Geometry check sheet. Reference: the model listing, model coordinates, mm. Coordinates: 2 decimals unless noted, no trailing zeros. Order: outer loops, then holes, each group sorted by start corner. A loop starts at its lowest first (then second) coordinate and runs counter-clockwise, first axis right, second up. Notation, with made-up numbers: (41.25, 50.5) - (90.25, 50.5) arc R12 ccw to (90.25, 64.5) - close; hole circle Ø9 at (68, 40). An arc over 180 degrees is marked (long way). Put each result on its own line as item: value.
from build123d import *

# Parameters (mm, degrees)
SKETCH2_W             = 2
SKETCH2_H             = 12
CUT_EXTRUDE1_DEPTH    = 10
SKETCH4_R             = 1.25
CUT_EXTRUDE2_DEPTH    = 10
CRVPATTERN2_OUTLINE_R = 1.25
CRVPATTERN2_DEPTH     = 2
SKETCH7_R             = 1.6
CUT_EXTRUDE3_DEPTH    = 2
SKETCH8_R             = 1.6
CUT_EXTRUDE4_DEPTH    = 11


# Read off the part's stored shape, not the designer's step: CrvPattern2
with BuildPart() as part:
    # Sweep1: sweep along a path in Sketch1
    with BuildLine(Plane(origin=(0, 0, 0), x_dir=(0, 0, -1), z_dir=(1, 0, 0))) as sweep1_path:
        ThreePointArc((0, 163.5), (-72.196731601, 108.101499399), (-37.371778265, 24.026624746))
        ThreePointArc((-37.371778265, 24.026624746), (-27.216931784, 13.871778265), (-23.5, 0))
    # Sketch2 → Sweep1 (sweep)
    with BuildSketch(Plane(origin=(0, 0, 0), x_dir=(1, 0, 0), z_dir=(0, 1, 0))):
        with Locations((1, -29.5)):
            Rectangle(SKETCH2_W, SKETCH2_H)
    sweep(path=sweep1_path.line)

    # Sketch3 → Cut-Extrude1 (cut)
    with BuildSketch(Plane(origin=(2, 0, 0), x_dir=(0, 0, -1), z_dir=(1, 0, 0))):
        with BuildLine():
            Line((0, 88.75644347), (-15.062860516, 174.182170465))
            ThreePointArc((-15.062860516, 174.182170465), (-7.560199098, 175.169914579), (0, 175.5))
            Line((0, 175.5), (0, 88.75644347))
        make_face()
    extrude(amount=-CUT_EXTRUDE1_DEPTH, mode=Mode.SUBTRACT)

    # Sketch4 → Cut-Extrude2 (cut)
    with BuildSketch(Plane.ZY):
        with Locations((26.912638139, 4.5)):
            Circle(SKETCH4_R)
    extrude(amount=-CUT_EXTRUDE2_DEPTH, mode=Mode.SUBTRACT)

    # CrvPattern2 outline → CrvPattern2 (cut)
    with BuildSketch(Plane.YZ):
        with Locations((18.911112769, 35.286946502)):
            Circle(CRVPATTERN2_OUTLINE_R)
        with Locations((12.43190695, 29.849835971)):
            Circle(CRVPATTERN2_OUTLINE_R)
        with Locations((161.000106646, 28.721311128)):
            Circle(CRVPATTERN2_OUTLINE_R)
        with Locations((157.434782313, 36.432764864)):
            Circle(CRVPATTERN2_OUTLINE_R)
        with Locations((153.049302567, 43.709139217)):
            Circle(CRVPATTERN2_OUTLINE_R)
        with Locations((147.896038722, 50.463539862)):
            Circle(CRVPATTERN2_OUTLINE_R)
        with Locations((142.036530957, 56.615305875)):
            Circle(CRVPATTERN2_OUTLINE_R)
        with Locations((135.540753402, 62.090972984)):
            Circle(CRVPATTERN2_OUTLINE_R)
        with Locations((128.486278509, 66.825150876)):
            Circle(CRVPATTERN2_OUTLINE_R)
        with Locations((120.957350684, 70.76130409)):
            Circle(CRVPATTERN2_OUTLINE_R)
        with Locations((113.043880237, 73.852427158)):
            Circle(CRVPATTERN2_OUTLINE_R)
        with Locations((104.840369684, 76.061605948)):
            Circle(CRVPATTERN2_OUTLINE_R)
        with Locations((96.44478519, 77.362458489)):
            Circle(CRVPATTERN2_OUTLINE_R)
        with Locations((87.957386665, 77.739450025)):
            Circle(CRVPATTERN2_OUTLINE_R)
        with Locations((79.479530462, 77.188078529)):
            Circle(CRVPATTERN2_OUTLINE_R)
        with Locations((71.112458978, 75.714928469)):
            Circle(CRVPATTERN2_OUTLINE_R)
        with Locations((62.956091619, 73.337592177)):
            Circle(CRVPATTERN2_OUTLINE_R)
        with Locations((55.107831572, 70.084459755)):
            Circle(CRVPATTERN2_OUTLINE_R)
        with Locations((47.661402606, 65.994380051)):
            Circle(CRVPATTERN2_OUTLINE_R)
        with Locations((40.705729836, 61.116196717)):
            Circle(CRVPATTERN2_OUTLINE_R)
        with Locations((34.323877772, 55.508164926)):
            Circle(CRVPATTERN2_OUTLINE_R)
        with Locations((28.592058371, 49.237255687)):
            Circle(CRVPATTERN2_OUTLINE_R)
        with Locations((23.578720911, 42.378356079)):
            Circle(CRVPATTERN2_OUTLINE_R)
    extrude(amount=CRVPATTERN2_DEPTH, mode=Mode.SUBTRACT)

    # Sketch7 → Cut-Extrude3 (cut)
    with BuildSketch(Plane.ZY):
        with Locations((35.390452374, 10)):
            Circle(SKETCH7_R)
        with Locations((76.299174561, 54.239502389)):
            Circle(SKETCH7_R)
        with Locations((79.721620809, 114.397161787)):
            Circle(SKETCH7_R)
        with Locations((41.871778265, 161.280490828)):
            Circle(SKETCH7_R)
    extrude(amount=-CUT_EXTRUDE3_DEPTH, mode=Mode.SUBTRACT)

    # Sketch8 → Cut-Extrude4 (cut)
    with BuildSketch(Plane(origin=(2, 0, 0), x_dir=(0, 0, -1), z_dir=(1, 0, 0))):
        with Locations((-19.266049694, 169.225788418)):
            Circle(SKETCH8_R)
    extrude(amount=-CUT_EXTRUDE4_DEPTH, mode=Mode.SUBTRACT)


solid = part.part
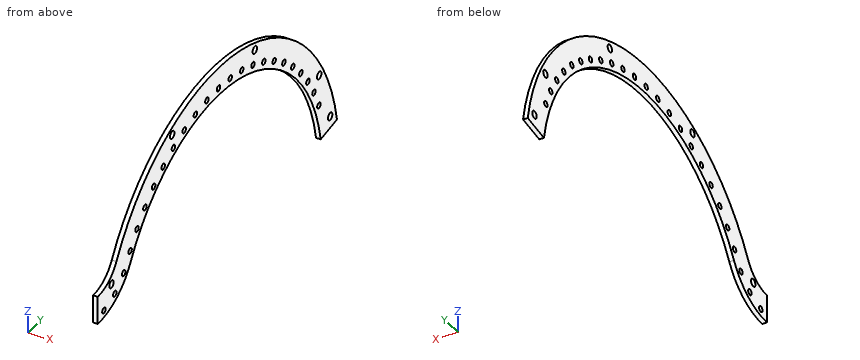
Q1. Section check B-B on x = 1.05. State how many separate pieces and enclosed holes the cut face has, then the cut area to 3 significant figures.
Answer block:
separate pieces: 1
enclosed holes: 29
area: 2,480 mm^2
Q2. Depth check by flat-ended pin: pin 1 Ø1 at (x, y) = (1.5, 65.5) entering from -Z. Enter the tip coordinate at first touch or a pass-through.
Answer block:
pin 1: stops at z = 70.87
Q3. Section check A-A on y = 100. Record the boundary of the cut face in (x, z), then the cut area to 3 significant figures.
Answer block:
outline: (0, 73.89) - (2, 73.89) - (2, 86.01) - (0, 86.01) - close
area: 24.2 mm^2
Q4. Section check C-C on y = 44. Record the boundary of the cut face in (x, z).
Answer block:
outline: (0, 59.86) - (2, 59.86) - (2, 74.31) - (0, 74.31) - close
Q5. Thickness scan on L1, parallel to Y at x = 0.8, z = 49; L2, parallel to Z at x = 1.55, y = 115; L3, parallel to Y at x = 1.75, z = 62.5. Record the ranges inside material, lowest first. Write a range as [from, to].
Answer block:
L1: y = [17.18, 27.36], [29.82, 32.32], [145.2, 160.33]
L2: z = [69.98, 78.24], [81.2, 82.68]
L3: y = [28.61, 47.76], [129.75, 134.36], [136.72, 148.91]
